from build123d import *

# Parameters (mm, degrees)
SKETCH1_R           = 1.5
BOSS_EXTRUDE1_DEPTH = 8.13
CUT_EXTRUDE1_DEPTH  = 16.25
CUT_EXTRUDE2_REACH  = 32.018
SKETCH3_W           = 13.5
SKETCH3_H           = 5.2
SKETCH4_R           = 1.5
CUT_EXTRUDE3_DEPTH  = 5.13
CUT_EXTRUDE4_REACH  = 96.714
SKETCH5_W           = 48.91393719
SKETCH5_H           = 4.31806182
FILLET1_R           = 1
CUT_EXTRUDE6_REACH  = 96.417
SKETCH8_R           = 1.875


with BuildPart() as part:
    # Sketch1 → Boss-Extrude1 (new body)
    with BuildSketch(Plane.XY):
        with BuildLine():
            Line((-24.456968595, 69.43193818), (24.456968595, 69.43193818))
            Line((24.456968595, 69.43193818), (23.121499045, 86.400687699))
            ThreePointArc((23.121499045, 86.400687699), (22.608100633, 87.588503122), (21.474960733, 88.213385013))
            Line((21.474960733, 88.213385013), (0, 92))
            Line((0, 92), (-21.474960733, 88.213385013))
            ThreePointArc((-21.474960733, 88.213385013), (-22.608100633, 87.588503122), (-23.121499045, 86.400687699))
            Line((-23.121499045, 86.400687699), (-24.456968595, 69.43193818))
        make_face()
        with Locations((-16, 81)):
            Circle(SKETCH1_R, mode=Mode.SUBTRACT)
        with Locations((16, 81)):
            Circle(SKETCH1_R, mode=Mode.SUBTRACT)
    extrude(amount=BOSS_EXTRUDE1_DEPTH)

    # Sketch2 → Cut-Extrude1 (cut)
    with BuildSketch(Plane(origin=(0, 92, 0), x_dir=(1, 0, 0), z_dir=(0, 1, 0))):
        Polygon((7.875, 0), (-4.875, 0), (-7.875, -2.565), (-7.875, -5.565), (-4.875, -8.13), (7.875, -8.13), align=None)
    extrude(amount=-CUT_EXTRUDE1_DEPTH, mode=Mode.SUBTRACT)

    # Sketch3 → Cut-Extrude2 (cut, up to next)
    with BuildSketch(Plane(origin=(0, 75.75, 0), x_dir=(1, 0, 0), z_dir=(0, 1, 0)), mode=Mode.PRIVATE) as cut_extrude2_sk1:
        with Locations((0, -4.065)):
            Rectangle(SKETCH3_W, SKETCH3_H)
    cut_extrude2_tool1 = extrude(cut_extrude2_sk1.sketch, amount=-CUT_EXTRUDE2_REACH, mode=Mode.PRIVATE) & part.part
    add(cut_extrude2_tool1.solids().sort_by_distance((0, 75.75, 4.065))[0], mode=Mode.SUBTRACT)

    # Sketch4 → Cut-Extrude3 (cut)
    # profile 1 of 2: a face of its own
    with BuildSketch(Plane(origin=(0, 0, 0), x_dir=(-1, 0, 0), z_dir=(0, 0, -1))):
        with BuildLine():
            Line((-10, 69.43193818), (-10, 90.236730193))
            Line((-10, 90.236730193), (-21.474960733, 88.213385013))
            ThreePointArc((-21.474960733, 88.213385013), (-22.608100633, 87.588503122), (-23.121499045, 86.400687699))
            Line((-23.121499045, 86.400687699), (-24.456968595, 69.43193818))
            Line((-24.456968595, 69.43193818), (-10, 69.43193818))
        make_face()
        with Locations(Location((-16, 81, 0), (0, 0, 180))):
            Circle(SKETCH4_R, mode=Mode.SUBTRACT)
    # profile 2 of 2: a face of its own
    with BuildSketch(Plane(origin=(0, 0, 0), x_dir=(-1, 0, 0), z_dir=(0, 0, -1))):
        with BuildLine():
            Line((10, 90.236730193), (10, 69.43193818))
            Line((10, 69.43193818), (24.456968595, 69.43193818))
            Line((24.456968595, 69.43193818), (23.121499045, 86.400687699))
            ThreePointArc((23.121499045, 86.400687699), (22.608100633, 87.588503122), (21.474960733, 88.213385013))
            Line((21.474960733, 88.213385013), (10, 90.236730193))
        make_face()
        with Locations(Location((16, 81, 0), (0, 0, 180))):
            Circle(SKETCH4_R, mode=Mode.SUBTRACT)
    extrude(amount=-CUT_EXTRUDE3_DEPTH, mode=Mode.SUBTRACT)

    # Sketch5 → Cut-Extrude4 (cut, up to next)
    with BuildSketch(Plane(origin=(0, 0, 0), x_dir=(-1, 0, 0), z_dir=(0, 0, -1)), mode=Mode.PRIVATE) as cut_extrude4_sk1:
        with Locations((0, 71.59096909)):
            Rectangle(SKETCH5_W, SKETCH5_H)
    cut_extrude4_tool1 = extrude(cut_extrude4_sk1.sketch, amount=-CUT_EXTRUDE4_REACH, mode=Mode.PRIVATE) & part.part
    add(cut_extrude4_tool1.solids().sort_by_distance((0, 71.590969, 0))[0], mode=Mode.SUBTRACT)

    # Fillet1
    # the kernel refuses this fillet: 1 mm, written as the material it adds along each edge
    with BuildSketch(Plane(origin=(-10, 92.736730193, 5.13), x_dir=(-1, 0, 0), z_dir=(0, -1, 0))) as fillet1_piece_1_section:
        with BuildLine():
            CenterArc((FILLET1_R, FILLET1_R), FILLET1_R, 180, 90)
            Line((0, FILLET1_R), (0, 0))
            Line((0, 0), (FILLET1_R, 0))
        make_face()
    fillet1_piece_1 = extrude(amount=18.986730193, mode=Mode.PRIVATE)
    fillet1_piece_1 = split(fillet1_piece_1, bisect_by=Plane(origin=(-11.632189481, 89.94893115, 4.903310521), z_dir=(0.17364817766693327, -0.9848077530122076, 0)), keep=Keep.TOP, mode=Mode.PRIVATE)
    add(fillet1_piece_1)
    with BuildSketch(Plane(origin=(6.75, 75.75, 1.465), x_dir=(0, 0, 1), z_dir=(0, -1, 0)), Plane(origin=(-6.75, 75.75, 6.665), x_dir=(0, 0, -1), z_dir=(0, -1, 0)), Plane(origin=(6.75, 75.75, 6.665), x_dir=(-1, 0, 0), z_dir=(0, -1, 0))) as fillet1_piece_2:
        with BuildLine():
            CenterArc((FILLET1_R, FILLET1_R), FILLET1_R, 180, 90)
            Line((0, FILLET1_R), (0, 0))
            Line((0, 0), (FILLET1_R, 0))
        make_face()
    extrude(amount=2)
    with BuildSketch(Plane(origin=(-6.75, 75.75, 1.465), x_dir=(0, 0, 1), z_dir=(0, -1, 0))) as fillet1_piece_3:
        with BuildLine():
            CenterArc((FILLET1_R, -FILLET1_R), FILLET1_R, 90, 90)
            Line((0, -FILLET1_R), (0, 0))
            Line((0, 0), (FILLET1_R, 0))
        make_face()
    extrude(amount=2)
    with BuildSketch(Plane(origin=(10, 73.75, 5.13), x_dir=(0, 0, -1), z_dir=(0, 1, 0))) as fillet1_piece_4_section:
        with BuildLine():
            CenterArc((FILLET1_R, -FILLET1_R), FILLET1_R, 90, 90)
            Line((0, -FILLET1_R), (0, 0))
            Line((0, 0), (FILLET1_R, 0))
        make_face()
    fillet1_piece_4 = extrude(amount=18.986730193, mode=Mode.PRIVATE)
    fillet1_piece_4 = split(fillet1_piece_4, bisect_by=Plane(origin=(11.632189481, 89.94893115, 4.903310521), z_dir=(-0.17364817766693252, -0.9848077530122077, 0)), keep=Keep.TOP, mode=Mode.PRIVATE)
    add(fillet1_piece_4)

    # Sketch8 → Cut-Extrude6 (cut, up to next)
    with BuildSketch(Plane(origin=(0, 0, 5.13), x_dir=(-1, 0, 0), z_dir=(0, 0, -1)), mode=Mode.PRIVATE) as cut_extrude6_sk1:
        with Locations((16, 81)):
            Circle(SKETCH8_R)
    cut_extrude6_tool1 = extrude(cut_extrude6_sk1.sketch, amount=-CUT_EXTRUDE6_REACH, mode=Mode.PRIVATE) & part.part
    # Sketch8 → Cut-Extrude6 (cut, up to next)
    with BuildSketch(Plane(origin=(0, 0, 5.13), x_dir=(-1, 0, 0), z_dir=(0, 0, -1)), mode=Mode.PRIVATE) as cut_extrude6_sk2:
        with Locations((-16, 81)):
            Circle(SKETCH8_R)
    cut_extrude6_tool2 = extrude(cut_extrude6_sk2.sketch, amount=-CUT_EXTRUDE6_REACH, mode=Mode.PRIVATE) & part.part
    add(cut_extrude6_tool1.solids().sort_by_distance((-16, 81, 5.13))[0], mode=Mode.SUBTRACT)
    add(cut_extrude6_tool2.solids().sort_by_distance((16, 81, 5.13))[0], mode=Mode.SUBTRACT)


solid = part.part
Input: part model. Units: mm. Frame: model coordinates. A direction names the side the tool comes from. Give positions to 0.01 mm unless a question says otherwise; leave off trailing zeros. Loops run counter-clockwise (first coordinate to the right, second up) from the corner with the lowest first, then second, coordinate; pieces in that order, holes last. Notation, with made-up numbers: M 71.25,55 L 128.25,55 A15 cw 128.25,78 Z; hole C -35,61.25 d4. An arc over 180 degrees is marked long. Use CSV: the item, a comma, the result in double quotes.
(1) Set-up query: faces 1 (the face through (-15.59, 79.17, 6.61)), 2 (the face through (-19, 82, 5.13)), 3 (the face through (7.875, 83, 4)), 4 (the face through (-22.6, 87.6, 6.6)), 5 (the face through (6.75, 75, 4)). Return all of +Z, -Z, +X, -X, +Y, -Y with unobstructed straight access to the full face (end or side cutting, diameter ignored); none if empty.
Outcome:
face 1,"+Z, -Z"
face 2,"-Z, -X, +Y, -Y"
face 3,"+Z, -Z, +Y"
face 4,"+Z, -Z, -X, +Y"
face 5,"+Y, -Y"
(2) Pull-direction query (X, two-part tool) for faces 6 (the face through (18, 82, 5.13)), 7 (the face through (6.465, 74.764, 6.364)), 8 (the face through (0, 75.75, 1)), 9 (the face through (10.285, 81.878, 4.829)); classes: pulls with the +X half, pulls with the -X half, needs draft (parallel to the pull), parting line crosses it, or undercut.
Outcome:
face 6,"needs draft"
face 7,"undercut"
face 8,"undercut"
face 9,"pulls with the +X half"
(3) Pin query (flat end, axial travel): P1, Ø1.5, axis at y = 85.5, z = 3.5, coming from the +X side; P2, Ø6.5, axis at x = 15.5, y = 82, coming from the -Z side; P3, Ø2, axis at y = 81.5, z = 2.5, coming from the -X side. Return the tip coordinate at first contact, or that it passes through.
Outcome:
P1,"stops at x = 10.01"
P2,"stops at z = 5.13"
P3,"stops at x = -10"
(4) Material intervals for L1, parallel to X at y = 81, z = 6.5 (3 decimals); L2, parallel to X at y = 81, z = 6.8 (3 decimals); L3, parallel to Z at x = 3.5, y = 74.5 (3 decimals), sorted ascending. Write a range as [from, to].
Outcome:
L1,"x = [-23.547, -17.875], [-14.125, -6.781], [7.875, 14.125], [17.875, 23.547]"
L2,"x = [-23.547, -17.875], [-14.125, -6.431], [7.875, 14.125], [17.875, 23.547]"
L3,"z = [0, 1.465], [6.665, 8.13]"
(5) Section A-A, the plane x = 2.5. Return loops of the section in (y, z) (3 decimals).
Outcome:
outline,"M 73.75,0 L 75.75,0 L 75.75,1.465 L 73.75,1.465 Z; M 73.75,6.665 L 75.75,6.665 L 75.75,8.13 L 73.75,8.13 Z"
(6) Section C-C, the plane y = 75.25. Return loops of the section in (x, z) (3 decimals), plus the area to 3 significant figures.
Outcome:
outline,"M -23.999,5.13 L -11,5.13 A1 cw -10,4.13 L -10,0 L 10,0 L 10,4.13 A1 cw 11,5.13 L 23.999,5.13 L 23.999,8.13 L -23.999,8.13 Z; hole M -6.75,2.465 A1 ccw -5.75,1.465 L 5.75,1.465 A1 ccw 6.75,2.465 L 6.75,5.665 A1 ccw 5.75,6.665 L -5.75,6.665 A1 ccw -6.75,5.665 Z"
area,"178 mm²"
(7) Section B-B, the plane y = 81.75. Return loops of the section in (x, z) (3 decimals).
Outcome:
outline,"M -23.488,5.13 L -17.718,5.13 L -17.718,8.13 L -23.488,8.13 Z; M -14.282,5.13 L -11,5.13 A1 cw -10,4.13 L -10,0 L -4.875,0 L -7.875,2.565 L -7.875,5.565 L -4.875,8.13 L -14.282,8.13 Z; M 7.875,0 L 10,0 L 10,4.13 A1 cw 11,5.13 L 14.282,5.13 L 14.282,8.13 L 7.875,8.13 Z; M 17.718,5.13 L 23.488,5.13 L 23.488,8.13 L 17.718,8.13 Z"
(8) Section D-D, the plane z = 7.5. Count the separate pieces of the cut face and the enclosed holes in it, plus the area to 3 significant figures.
Outcome:
separate pieces,"1"
enclosed holes,"2"
area,"528 mm²"
